from build123d import *

# Parameters (mm, degrees)
SKETCH_1_R          = 5.5
EXTRUDE_1_DEPTH     = 6
CUT_EXTRUDE_4_DEPTH = 10.823441352
SKETCH_3_R          = 3.5
EXTRUDE_5_DEPTH     = 27


with BuildPart() as part:
    # Эскиз1 → Вытянуть1 (new body)
    with BuildSketch(Plane(origin=(0, 0, 0), x_dir=(1, 0, 0), z_dir=(0, 1, 0))):
        with Locations(Location((0, 0, 0), (0, 0, 270))):
            Circle(SKETCH_1_R)
    extrude(amount=EXTRUDE_1_DEPTH)

    # Эскиз2 → Вытянуть4 (cut, through all)
    with BuildSketch(Plane(origin=(0, 0, 0), x_dir=(1, 0, 0), z_dir=(0, 1, 0))):
        Polygon((-0.5, 5.758821463), (0.5, 5.758821463), (0, 4.437090717), align=None)
        Polygon((0.669477267, 5.741587309), (0.893179795, 4.346263209), (1.649007209, 5.540288789), align=None)
        Polygon((1.811546057, 5.489291897), (1.749792704, 4.077499175), (2.730503868, 5.094936042), align=None)
        Polygon((2.879449938, 5.012264229), (2.534768894, 3.641801846), (3.700213379, 4.440996014), align=None)
        Polygon((3.8294688, 4.330033874), (3.215971348, 3.057008721), (4.518435719, 3.605241087), align=None)
        Polygon((4.622708759, 3.470531425), (3.765511557, 2.3470613), (5.15167277, 2.621887167), align=None)
        Polygon((5.226694479, 2.46894501), (4.16089128, 1.541024913), (5.573999732, 1.531192878), align=None)
        Polygon((5.616698713, 1.366279697), (4.385923626, 0.671898786), (5.76812649, 0.377811373), align=None)
        Polygon((5.776754641, 0.207678733), (4.431395743, -0.224734957), (5.726105473, -0.791037774), align=None)
        Polygon((5.700309556, -0.959424623), (4.295445997, -1.112168024), (5.449657024, -1.927501742), align=None)
        Polygon((5.390493128, -2.087249022), (3.983640188, -1.954068802), (4.950098976, -2.985053562), align=None)
        Polygon((4.859989278, -3.129621201), (3.508743681, -2.715969773), (4.247883295, -3.920396938), align=None)
        Polygon((4.130516895, -4.043866321), (2.890198796, -3.366678623), (3.371758773, -4.695238804), align=None)
        Polygon((3.231940666, -4.792555078), (2.153328833, -3.879555254), (2.35759405, -5.27785704), align=None)
        Polygon((2.201048406, -5.345036067), (1.328301334, -4.233602437), (1.24690915, -5.64439919), align=None)
        Polygon((1.080044966, -5.678690651), (0.448893022, -4.414325439), (0.085175642, -5.779858973), align=None)
        Polygon((-0.085175642, -5.779858973), (-0.448893022, -4.414325439), (-1.080044966, -5.678690651), align=None)
        Polygon((-1.24690915, -5.64439919), (-1.328301334, -4.233602437), (-2.201048406, -5.345036067), align=None)
        Polygon((-2.35759405, -5.27785704), (-2.153328833, -3.879555254), (-3.231940666, -4.792555078), align=None)
        Polygon((-3.371758773, -4.695238804), (-2.890198796, -3.366678623), (-4.130516895, -4.043866321), align=None)
        Polygon((-4.247883295, -3.920396938), (-3.508743681, -2.715969773), (-4.859989278, -3.129621201), align=None)
        Polygon((-4.950098976, -2.985053562), (-3.983640188, -1.954068802), (-5.390493128, -2.087249022), align=None)
        Polygon((-5.449657024, -1.927501742), (-4.295445997, -1.112168024), (-5.700309556, -0.959424623), align=None)
        Polygon((-5.726105473, -0.791037774), (-4.431395743, -0.224734957), (-5.776754641, 0.207678733), align=None)
        Polygon((-5.76812649, 0.377811373), (-4.385923626, 0.671898786), (-5.616698713, 1.366279697), align=None)
        Polygon((-5.573999732, 1.531192878), (-4.16089128, 1.541024913), (-5.226694479, 2.46894501), align=None)
        Polygon((-5.15167277, 2.621887167), (-3.765511557, 2.3470613), (-4.622708759, 3.470531425), align=None)
        Polygon((-4.518435719, 3.605241087), (-3.215971348, 3.057008721), (-3.8294688, 4.330033874), align=None)
        Polygon((-3.700213379, 4.440996014), (-2.534768894, 3.641801846), (-2.879449938, 5.012264229), align=None)
        Polygon((-2.730503868, 5.094936042), (-1.749792704, 4.077499175), (-1.811546057, 5.489291897), align=None)
        Polygon((-1.649007209, 5.540288789), (-0.893179795, 4.346263209), (-0.669477267, 5.741587309), align=None)
    extrude(amount=CUT_EXTRUDE_4_DEPTH, mode=Mode.SUBTRACT)

    # Эскиз3 → Вытянуть5 (add)
    with BuildSketch(Plane(origin=(0, 6, 0), x_dir=(-1, 0, 0), z_dir=(0, 1, 0))):
        with Locations(Location((0, 0, 0), (0, 0, 90))):
            Circle(SKETCH_3_R)
    extrude(amount=EXTRUDE_5_DEPTH)


solid = part.part
Check sheet for the modelled part. Datum: model origin and axes. Units: mm. Give positions to 0.01 mm unless a question says otherwise; leave off trailing zeros. Loops run counter-clockwise (first coordinate to the right, second up) from the corner with the lowest first, then second, coordinate; pieces in that order, holes last. Notation, with made-up numbers: M 44,4.5 L 54,4.5 A21 ccw 54,35.5 Z; hole C 52.25,46 d3. An arc over 180 degrees is marked long. Return JSON: item names as keys, results as strings. Group by question number.
1. Cross-section at A-A on y = 22. Record the boundary of the cut face in (x, z).
2. Go/stop test with flat-tipped pins: pin 1 (6 mm diameter, centred on y = 11, z = 4, fed in from -X); pin 2 (4 mm diameter, centred on x = -2, y = 18.5, fed in from +Z); pin 3 (3 mm diameter, centred on y = 14, z = 4, fed in from -X). Record where each tip stops, or that it passes through.
3. Thickness scan on L1, parallel to Y at x = 3.75, z = -1.75; L2, parallel to X at y = 10, z = 0.5; L3, parallel to Z at x = 2.5, y = 19. Record the ranges inside material, lowest first.
Return value:
{
 "1": {"outline": "C 0,0 d7"},
 "2": {"pin 1": "x = -3.35", "pin 2": "z = 3.5", "pin 3": "x = -2.45"},
 "3": {"L1": "0 to 6", "L2": "-3.46 to 3.46", "L3": "-2.45 to 2.45"}
}
